Input: part model. Units: mm. Frame: model coordinates. Face numbers are marked on the shaded views. A direction names the side the tool comes from. Coordinates: 2 decimals unless noted, no trailing zeros. Loops run counter-clockwise (first coordinate to the right, second up) from the corner with the lowest first, then second, coordinate; pieces in that order, holes last.
(1) Contact query for flat-ended pins moving along their axis: P1, Ø25, axis at y = 0, z = 0, coming from the -X side (3 decimals); P2, Ø10, axis at x = 42.5, z = -1.5, coming from the -Y side; P3, Ø19.5, axis at y = 0, z = 0, coming from the -X side; P4, Ø5, axis at x = 92.5, y = 25.5, coming from the -Z side. Output: stop coordinate, or through.
(2) Section C-C, the plane x = 151. Return loops of the section in (y, z) (3 decimals), then the cut area to 3 significant figures.
(3) Section A-A, the plane z = 0. Return loops of the section in (x, y) (3 decimals).
(4) Line query: L1, parallel to X at y = -10.5, z = 24; L2, parallel to Z at x = 78, y = 0 (3 decimals). Output: solid intervals per line, ascending.
(5) Set-up query: the marked faces 1, 2 and 3. Return all of +Z, -Z, +X, -X, +Y, -Y with unobstructed straight access to the full face (end or side cutting, diameter ignored); none if empty.
(6) Section D-D, the plane y = -23. Return loops of the section in (x, z), then the cut area to 3 significant figures.
(7) Mould query, pull axis X, two halves, no side actions, for the marked faces 4, 5, 6 and 7. Classes: released by +X, released by -X, zero draft, split by the parting line, or undercut.
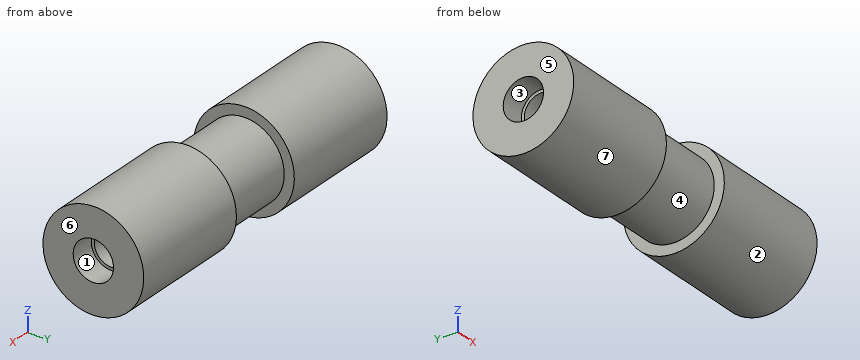
```python
from build123d import *

# Parameters (mm, degrees)
SKETCH1_R           = 31.75
SKETCH1_R_2         = 10.795
BOSS_EXTRUDE1_DEPTH = 106.68
SKETCH2_R           = 12.7
CUT_EXTRUDE1_DEPTH  = 15.875
CUT_EXTRUDE2_START  = -81.28
SKETCH3_OUTSIDE_W   = 111.798
SKETCH3_OUTSIDE_H   = 111.798
SKETCH3_OUTSIDE_R   = 25.4
CUT_EXTRUDE2_DEPTH  = 50.8


with BuildPart() as part:
    # Sketch1 → Boss-Extrude1 (new body)
    with BuildSketch(Plane(origin=(0, 0, 0), x_dir=(0, 0, -1), z_dir=(1, 0, 0))):
        Circle(SKETCH1_R)
        Circle(SKETCH1_R_2, mode=Mode.SUBTRACT)
    boss_extrude1 = extrude(amount=BOSS_EXTRUDE1_DEPTH)

    # Sketch2 → Cut-Extrude1 (cut)
    with BuildSketch(Plane.ZY):
        Circle(SKETCH2_R)
    cut_extrude1 = extrude(amount=-CUT_EXTRUDE1_DEPTH, mode=Mode.SUBTRACT)

    # Mirror1: Boss-Extrude1, Cut-Extrude1 across plane
    add(boss_extrude1.mirror(Plane(origin=(106.68, 0, 0), x_dir=(0, 0, 1), z_dir=(1, 0, 0))))
    add(cut_extrude1.mirror(Plane(origin=(106.68, 0, 0), x_dir=(0, 0, 1), z_dir=(1, 0, 0))), mode=Mode.SUBTRACT)

    # Sketch3 outside → Cut-Extrude2 (cut)
    with BuildSketch(Plane.ZY.offset(CUT_EXTRUDE2_START)):
        Rectangle(SKETCH3_OUTSIDE_W, SKETCH3_OUTSIDE_H)
        Circle(SKETCH3_OUTSIDE_R, mode=Mode.SUBTRACT)
    extrude(amount=-CUT_EXTRUDE2_DEPTH, mode=Mode.SUBTRACT)


solid = part.part
```
Report:
1. P1: stops at x = 15.875
1. P2: stops at y = -31.75
1. P3: passes through
1. P4: stops at z = -10.78
2. outline: circle Ø63.5 at (0, 0); hole circle Ø21.59 at (0, 0)
2. area: 2,800 mm2
3. outline: (0, -31.75) - (81.28, -31.75) - (81.28, -25.4) - (132.08, -25.4) - (132.08, -31.75) - (213.36, -31.75) - (213.36, -12.7) - (197.485, -12.7) - (197.485, -10.795) - (15.875, -10.795) - (15.875, -12.7) - (0, -12.7) - close; (0, 12.7) - (15.875, 12.7) - (15.875, 10.795) - (197.485, 10.795) - (197.485, 12.7) - (213.36, 12.7) - (213.36, 31.75) - (132.08, 31.75) - (132.08, 25.4) - (81.28, 25.4) - (81.28, 31.75) - (0, 31.75) - close
4. L1: x = 0 to 81.28, 132.08 to 213.36
4. L2: z = -31.75 to -10.795, 10.795 to 31.75
5. face 1: +X
5. face 2: +X, -X
5. face 3: -X
6. outline: (0, -21.89) - (81.28, -21.89) - (81.28, -10.78) - (132.08, -10.78) - (132.08, -21.89) - (213.36, -21.89) - (213.36, 21.89) - (132.08, 21.89) - (132.08, 10.78) - (81.28, 10.78) - (81.28, 21.89) - (0, 21.89) - close
6. area: 8,210 mm2
7. face 4: undercut
7. face 5: released by -X
7. face 6: released by +X
7. face 7: zero draft
